from build123d import *

# Parameters (mm, degrees)
SKETCH_1_R               = 100
EXTRUDE_1_DEPTH          = 10
CUT_EXTRUDE_5_DEPTH      = 142.774468788
PATTERN_CIRCULAR_1_COUNT = 8


with BuildPart() as part:
    # 草圖1 → 伸長1 (new body)
    with BuildSketch(Plane.XY):
        Circle(SKETCH_1_R)
    extrude(amount=EXTRUDE_1_DEPTH)

    # 草圖2 → 伸長5 (cut, through all)
    with BuildSketch(Plane.XY):
        with BuildLine():
            ThreePointArc((14.160251472, 95.254255396), (11.972243623, 88.027756377), (14.160251472, 80.801257358))
            ThreePointArc((14.160251472, 80.801257358), (13.535533906, 74.492222471), (7.226499019, 73.867504906))
            ThreePointArc((7.226499019, 73.867504906), (0, 76.055512755), (-7.226499019, 73.867504906))
            ThreePointArc((-7.226499019, 73.867504906), (-13.535533906, 74.492222471), (-14.160251472, 80.801257358))
            ThreePointArc((-14.160251472, 80.801257358), (-11.972243623, 88.027756377), (-14.160251472, 95.254255396))
            ThreePointArc((-14.160251472, 95.254255396), (-13.535533906, 101.563290283), (-7.226499019, 102.188007849))
            ThreePointArc((-7.226499019, 102.188007849), (0, 100), (7.226499019, 102.188007849))
            ThreePointArc((7.226499019, 102.188007849), (13.535533906, 101.563290283), (14.160251472, 95.254255396))
        make_face()
    cut_extrude_5 = extrude(amount=CUT_EXTRUDE_5_DEPTH, mode=Mode.SUBTRACT)

    # 環狀複製排列1: 伸長5 ×8 about axis
    pattern_circular_1_axis = Axis((0, 0, 0), (0, 0, 1))
    for i in range(1, PATTERN_CIRCULAR_1_COUNT):
        add(cut_extrude_5.rotate(pattern_circular_1_axis, i * 360 / PATTERN_CIRCULAR_1_COUNT), mode=Mode.SUBTRACT)


solid = part.part
Source: CAD feature listing. Evaluate the final solid. Frame: model axes, mm. A direction names the side the tool comes from. Coordinates: 2 decimals unless noted, no trailing zeros. Order: outer loops, then holes, each group sorted by start corner. A loop starts at its lowest first (then second) coordinate and runs counter-clockwise, first axis right, second up.
Item 1: Cut plane B-B (y = 55). Return loops of the section in (x, z), plus the area to 3 significant figures.
Output values:
outline: (-83.52, 0) - (-72.12, 0) - (-72.12, 10) - (-83.52, 10) - close; (-52.37, 0) - (52.37, 0) - (52.37, 10) - (-52.37, 10) - close; (72.12, 0) - (83.52, 0) - (83.52, 10) - (72.12, 10) - close
area: 1,280 mm2
Item 2: Set-up query: faces 1 (the face through (43.104, 62.149, 4.93)), 2 (the face through (70.787, 53.855, 4.93)). Return all of +Z, -Z, +X, -X, +Y, -Y with unobstructed straight access to the full face (end or side cutting, diameter ignored); none if empty.
Output values:
face 1: +Z, -Z
face 2: +Z, -Z, +Y
Item 3: Cut plane D-D (x = -38.5). Return loops of the section in (y, z).
Output values:
outline: (-92.29, 0) - (92.29, 0) - (92.29, 10) - (-92.29, 10) - close
Item 4: Cut plane A-A (x = 49.5). Return loops of the section in (y, z), plus the area to 3 significant figures.
Output values:
outline: (-86.89, 0) - (-67.86, 0) - (-67.86, 10) - (-86.89, 10) - close; (-56.63, 0) - (56.63, 0) - (56.63, 10) - (-56.63, 10) - close; (67.86, 0) - (86.89, 0) - (86.89, 10) - (67.86, 10) - close
area: 1,510 mm2
Item 5: First-contact query: P1, Ø1.5, axis at x = 34.5, z = 5.5, coming from the +Y side; P2, Ø3, axis at x = -47.5, z = 6.5, coming from the +Y side; P3, Ø5, axis at x = -66, z = 6.5, coming from the +Y side. Flat tips, straight axial feed; report the tip coordinate or a pass-through.
Output values:
P1: stops at y = 94.13
P2: stops at y = 88.79
P3: stops at y = 50.83
Item 6: Cut plane C-C (y = -0.5). Return loops of the section in (x, z), plus the area to 3 significant figures.
Output values:
outline: (-76.05, 0) - (76.05, 0) - (76.05, 10) - (-76.05, 10) - close
area: 1,520 mm2
Item 7: Material intervals for line 1 (X direction, y = 48, z = 3.75); line 2 (X direction, y = -51.5, z = 6); line 3 (X direction, y = 85, z = 4.25), sorted ascending.
Output values:
line 1: x = -87.73 to -67.36, -57.13 to 57.13, 67.36 to 87.73
line 2: x = -85.72 to -68.89, -55.6 to 55.6, 68.89 to 85.72
line 3: x = -52.68 to -12.33, 12.33 to 52.68
Item 8: Pull-direction query (X, two-part tool) for faces 3 (the face through (-43.104, 62.341, 4.93)), 4 (the face through (-92.5, -38, 4.9)), 5 (the face through (92.26, -38.58, 4.93)); classes: pulls with the +X half, pulls with the -X half, needs draft (parallel to the pull), parting line crosses it, or undercut.
Output values:
face 3: undercut
face 4: pulls with the -X half
face 5: pulls with the +X half
